Part print with two shaded views. Sizes in mm from the minimum x, y, z corner. Coordinates: 2 decimals unless noted, no trailing zeros. Write each loop counter-clockwise with the first axis right and the second up, starting at its lowest first coordinate (ties: lowest second). Pieces come first, ordered by that corner, then holes. Notation, with made-up numbers: (13.25, 49.5) -> (17.25, 49.5) arc R25 ccw to (17.25, 64.5) -> close; hole circle Ø3 at (-5, -26.75). An arc over 180 degrees is marked (long way). Write item = value, one per line. Start each with the question number.
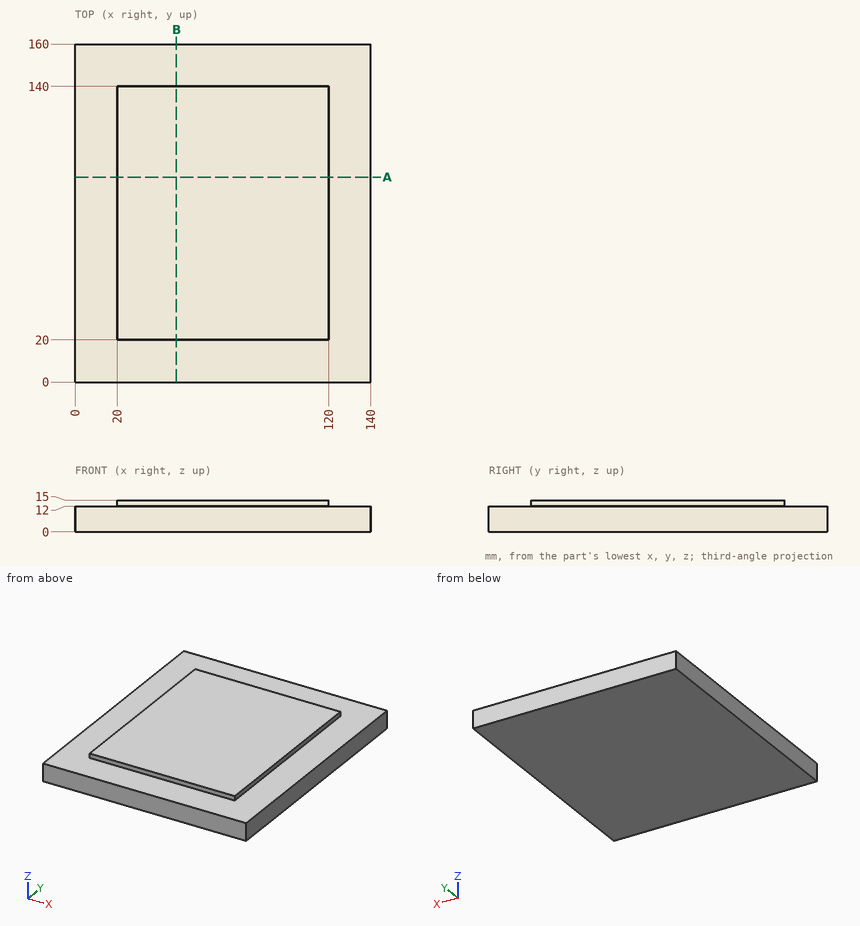
(1) Saw through at A-A (y = 97). Give the cut face in (x, z), then the cut area to 3 significant figures.
(2) Drill centre lines: line 1 along Z through (x, y) = (51, 13); line 2 along Y through (x, z) = (36, 12.5); line 3 along X through (y, z) = (96, 12.25). Where is each one in solid material? Low to high.
(3) Saw through at B-B (x = 48). Give the cut face in (y, z), then the cut area to 3 significant figures.
(4) Drop flat-ended pins along their axis: pin 1 Ø0.9 at (x, z) = (94.5, 14) entering from +Y; pin 2 Ø0.9 at (y, z) = (109.5, 14) entering from -X; pin 3 Ø0.9 at (x, z) = (74, 13.5) entering from -Y. Give the stop position or say it passes through.
Returned:
q1.outline = (0, 0) -> (140, 0) -> (140, 12) -> (120, 12) -> (120, 15) -> (20, 15) -> (20, 12) -> (0, 12) -> close
q1.area = 1,980 mm2
q2.line_1 = 0 to 12
q2.line_2 = 20 to 140
q2.line_3 = 20 to 120
q3.outline = (0, 0) -> (160, 0) -> (160, 12) -> (140, 12) -> (140, 15) -> (20, 15) -> (20, 12) -> (0, 12) -> close
q3.area = 2,280 mm2
q4.pin_1 = 140
q4.pin_2 = 20
q4.pin_3 = 20
